Geometry: final body of the model. Coordinates: model frame, mm. A direction names the side the tool comes from. Round coordinates to 2 decimals unless told otherwise and drop trailing zeros. Loops run counter-clockwise (first coordinate to the right, second up) from the corner with the lowest first, then second, coordinate; pieces in that order, holes last. Notation, with made-up numbers: (27.5, -36) - (75.5, -36) arc R24 ccw to (75.5, -4) - close; hole circle Ø11 at (15.5, 50.5). An arc over 180 degrees is marked (long way). Use CSV: the item, a comma, the result in double quotes.
Solid Edge part; units mm, degrees
sketch "Sketch1" plane through (0, 0, 0) normal (0, 0, 1) x (1, 0, 0)
  circle A0 centre (0, 0) radius 3.3
extrude "Protrusion1" add sketch "Sketch1" along normal blind 4.8
sketch "Sketch2" plane through (0, 0, 0) normal (0, 0, -1) x (1, 0, 0)
  circle A0 centre (0, 0) radius 2.25
extrude "Extrusionsausschnitt_1" cut sketch "Sketch2" against normal blind 0.8
sketch "Sketch3" plane through (0, 0, 0.8) normal (0, 0, -1) x (1, 0, 0)
  circle A0 centre (0, 0) radius 1.4
extrude "Cutout1" cut sketch "Sketch3" against normal through all
sketch "Sketch4" plane through (0, 0, 4.8) normal (0, 0, 1) x (1, 0, 0)
  circle A0 centre (0, 0) radius 2.2
extrude "Extrusionsausschnitt_3" cut sketch "Sketch4" against normal blind 2.8
sketch "Sketch5" plane through (0, 0, 2.4) normal (0, 0, 1) x (1, 0, 0)
  line L0 (-2.2108, 2.45) -> (-14.25, 1.8)
  arc A0 (-14.25, 1.8) -> (-14.25, -1.8) centre (-13.8578, 0) ccw
  line L1 (-14.25, -1.8) -> (-2.2108, -2.45)
  arc A1 (-2.2108, 2.45) -> (-2.2108, -2.45) centre (0, 0) ccw
  line L2 (2.2108, 2.45) -> (14.25, 1.8)
  arc A2 (14.25, 1.8) -> (14.25, -1.8) centre (13.8578, 0) cw
  line L3 (2.2108, -2.45) -> (14.25, -1.8)
  arc A3 (2.2108, 2.45) -> (2.2108, -2.45) centre (0, 0) cw
  dimension "D1" = 14.25
  dimension "D2" = 2.2108
extrude "Extrusionsausprägung_2" add sketch "Sketch5" against normal blind 2
sketch "Sketch6" plane through (0, 0, 0) normal (0, 0, 1) x (1, 0, 0)
  circle A0 centre (-14, 0) radius 0.6
  circle A1 centre (-12.1, 0) radius 0.6
  circle A2 centre (-10.2, 0) radius 0.6
  circle A3 centre (-8.3, 0) radius 0.6
  circle A4 centre (-6.4, 0) radius 0.6
  circle A5 centre (-4.5, 0) radius 0.6
  dimension "D1" = 14
extrude "Cutout2" cut sketch "Sketch6" along normal through all
mirror "Mirror1" about plane through (0, 0, 0) normal (1, 0, 0) of "Cutout2"
Item 1: Section B-B on y = 0. Give the number of separate pieces and of enclosed holes in the cut face, plus the area to 3 significant figures.
Final values:
separate pieces,"14"
enclosed holes,"0"
area,"33.2 mm²"
Item 2: Section A-A on x = 8. Return the cut outline in (y, z), plus the area to 3 significant figures.
Final values:
outline,"(-2.14, 0.4) - (-0.52, 0.4) - (-0.52, 2.4) - (-2.14, 2.4) - close; (0.52, 0.4) - (2.14, 0.4) - (2.14, 2.4) - (0.52, 2.4) - close"
area,"6.47 mm²"
Item 3: Mould query, pull axis Y, two halves, no side actions, for faces 3 (the flat face through (8.15, 2.13, 1.41)), 4 (the cylindrical face through (3.05, 1.26, 2.9)), 5 (the cylindrical face through (12.7, 0, 1.4)). Classes: released by +Y, released by -Y, zero draft, split by the parting line, or undercut.
Final values:
face 3,"released by +Y"
face 4,"split by the parting line"
face 5,"undercut"
Item 4: Pin query (flat end, axial travel): P1, Ø2, axis at y = 0, z = 2.5, coming from the +X side; P2, Ø1, axis at x = -12.1, y = 0, coming from the -Z side; P3, Ø1, axis at x = 6, y = 0, coming from the +Z side; P4, Ø2, axis at x = 7, y = -1, coming from the -Z side. Return the tip coordinate at first contact, or that it passes through.
Final values:
P1,"stops at x = 15.7"
P2,"passes through"
P3,"stops at z = 2.4"
P4,"stops at z = 0.4"
Item 5: Section D-D on y = -2.75. Return the cut outline in (x, z).
Final values:
outline,"(-1.82, 0) - (1.82, 0) - (1.82, 4.8) - (-1.82, 4.8) - close"
Item 6: Section C-C on x = -4.5. Return the cut outline in (y, z).
Final values:
outline,"(-2.33, 0.4) - (-0.6, 0.4) - (-0.6, 2.4) - (-2.33, 2.4) - close; (0.6, 0.4) - (2.33, 0.4) - (2.33, 2.4) - (0.6, 2.4) - close"
Item 7: Reachability of faces 1 (the cylindrical face through (7.728, 0.18, 1.386)), 2 (the cylindrical face through (2.1, 0.66, 3.42)) from +Z, -Z, +X, -X, +Y, -Y: full face, straight path, thin tool, end or side. Return the list, or none.
Final values:
face 1,"+Z, -Z"
face 2,"+Z"
Item 8: Material intervals for line 1 (Z direction, x = 8.5, y = 1.5); line 2 (X direction, y = -2, z = 3.5); line 3 (X direction, y = 0.25, z = 2.65), sorted ascending.
Final values:
line 1,"z = 0.4 to 2.4"
line 2,"x = -2.62 to -0.92, 0.92 to 2.62"
line 3,"x = -3.29 to -2.19, 2.19 to 3.29"
